The model under review builds one solid part; all positions refer to its coordinate system, in mm. A direction names the side the tool comes from. Give positions to 0.01 mm unless a question says otherwise; leave off trailing zeros. Order: outer loops, then holes, each group sorted by start corner. A loop starts at its lowest first (then second) coordinate and runs counter-clockwise, first axis right, second up.
```python
from build123d import *

# Parameters (mm, degrees)
SKETCH1_R           = 8.45
BOSS_EXTRUDE1_DEPTH = 13.6
BOSS_EXTRUDE2_DEPTH = 6.9
SKETCH3_R           = 6
BOSS_EXTRUDE3_DEPTH = 12
SKETCH5_R           = 6
SKETCH5_R_2         = 5.75
CUT_EXTRUDE1_DEPTH  = 1.1


with BuildPart() as part:
    # Sketch1 → Boss-Extrude1 (new body)
    with BuildSketch(Plane.XY):
        Circle(SKETCH1_R)
    extrude(amount=-BOSS_EXTRUDE1_DEPTH)

    # Sketch2 → Boss-Extrude2 (add)
    with BuildSketch(Plane.XY):
        Polygon((0, 13.221321164), (-11.45, 6.610660582), (-11.45, -6.610660582), (0, -13.221321164), (11.45, -6.610660582), (11.45, 6.610660582), align=None)
    extrude(amount=BOSS_EXTRUDE2_DEPTH)

    # Sketch3 → Boss-Extrude3 (add)
    with BuildSketch(Plane(origin=(0, 0, -13.6), x_dir=(-1, 0, 0), z_dir=(0, 0, -1))):
        Circle(SKETCH3_R)
    extrude(amount=BOSS_EXTRUDE3_DEPTH)

    # Sketch5 → Cut-Extrude1 (cut)
    with BuildSketch(Plane(origin=(0, 0, -21.9), x_dir=(-1, 0, 0), z_dir=(0, 0, -1))):
        Circle(SKETCH5_R)
        Circle(SKETCH5_R_2, mode=Mode.SUBTRACT)
    extrude(amount=CUT_EXTRUDE1_DEPTH, mode=Mode.SUBTRACT)


solid = part.part
```
1. For faces 4 (the cylindrical face through (6, 0, -24)), 5 (the flat face through (-11.45, 0, 3)), list the 3-axis set-ups (+Z, -Z, +X, -X, +Y, -Y) from which the entire face can be reached by the end or side of a thin tool; tool diameter is ignored.
2. To check wall thickness, follow line 1 (Z direction, x = 9, y = -1.25); line 2 (Z direction, x = 7.5, y = -2.5); line 3 (Y direction, x = -5.25, z = -7). State the ranges of each line that lie inside material, in increasing order.
3. Draft analysis for pull direction Z (two halves, no side actions). For faces 1 (the flat face through (-5.645, 9.962, 3.402)), 2 (the cylindrical face through (0.75, 5.7, -22.44)), 3 (the flat face through (0, -9, 0)), state which applies: pulls with the +Z half, pulls with the -Z half, needs draft (parallel to the pull), parting line crosses it, or undercut.
4. Take a section at A-A (y = 0). Write out the cut boundary in (x, z).
5. Take a section at B-B (z = 1.5). Write out the cut boundary in (x, y), and give its area (3 significant figures).
6. Take a section at D-D (y = -7.5). Write out the cut boundary in (x, z), and give its area (3 significant figures).
7. Take a section at C-C (x = -3). Write out the cut boundary in (y, z), and give its area (3 significant figures).
8. Insertion check: pin 1 (1.5 mm diameter, centred on y = -3, z = -22, fed in from -X); pin 2 (1 mm diameter, centred on y = -4, z = -18.5, fed in from -X); pin 3 (6 mm diameter, centred on y = -8.5, z = -3.5, fed in from -X) (3 decimals). Each pin has a flat end and moves straight along its axis. Give the tip position at first contact, or say it passes through.
Answer:
1. face 4: -Z
1. face 5: +Z, -Z, -X, +Y, -Y
2. line 1: z = 0 to 6.9
2. line 2: z = -13.6 to 6.9
2. line 3: y = -6.62 to 6.62
3. face 1: needs draft
3. face 2: undercut
3. face 3: pulls with the -Z half
4. outline: (-11.45, 0) - (-8.45, 0) - (-8.45, -13.6) - (-6, -13.6) - (-6, -21.9) - (-5.75, -21.9) - (-5.75, -23) - (-6, -23) - (-6, -25.6) - (6, -25.6) - (6, -23) - (5.75, -23) - (5.75, -21.9) - (6, -21.9) - (6, -13.6) - (8.45, -13.6) - (8.45, 0) - (11.45, 0) - (11.45, 6.9) - (-11.45, 6.9) - close
5. outline: (-11.45, -6.61) - (0, -13.22) - (11.45, -6.61) - (11.45, 6.61) - (0, 13.22) - (-11.45, 6.61) - close
5. area: 454 mm2
6. outline: (-9.91, 0) - (-3.89, 0) - (-3.89, -13.6) - (3.89, -13.6) - (3.89, 0) - (9.91, 0) - (9.91, 6.9) - (-9.91, 6.9) - close
6. area: 243 mm2
7. outline: (-11.49, 0) - (-7.9, 0) - (-7.9, -13.6) - (-5.2, -13.6) - (-5.2, -21.9) - (-4.91, -21.9) - (-4.91, -23) - (-5.2, -23) - (-5.2, -25.6) - (5.2, -25.6) - (5.2, -23) - (4.91, -23) - (4.91, -21.9) - (5.2, -21.9) - (5.2, -13.6) - (7.9, -13.6) - (7.9, 0) - (11.49, 0) - (11.49, 6.9) - (-11.49, 6.9) - close
7. area: 497 mm2
8. pin 1: stops at x = -5.56
8. pin 2: stops at x = -4.87
8. pin 3: stops at x = -6.415
